Model file for the job. Use its own axes, mm. A direction names the side the tool comes from. Give positions to 0.01 mm unless a question says otherwise; leave off trailing zeros. Loops run counter-clockwise (first coordinate to the right, second up) from the corner with the lowest first, then second, coordinate; pieces in that order, holes last. Notation, with made-up numbers: M -8,-28.5 L -1,-28.5 A14 cw -1,-2.5 Z; hole C 87,-17 d4. An arc over 180 degrees is marked long. Answer in a Markdown table with one row per item.
```python
from build123d import *

# Parameters (mm, degrees)
F0_W      = 12.9794
F0_H      = 25.908
F1_DEPTH  = 25.4889
F2_W      = 38.1
F2_H      = 12.7
F3_DEPTH  = 6.35
F6_W      = 37.945812
F6_H      = 12.68057
F7_DEPTH  = 12.7
F8_W      = 50.9778
F8_H      = 12.7
F9_DEPTH  = 50.8
F10_R     = 12.7
F11_DEPTH = 12.701
F12_R     = 25.4


with BuildPart() as f1:
    # F0 (on Right) → F1 (new body, symmetric)
    with BuildSketch(Plane.YZ):
        with Locations((30.203413, 4.414101)):
            Rectangle(F0_W, F0_H)
    extrude(amount=F1_DEPTH, both=True)

    # F6 (on face) → F7 (join)
    with BuildSketch(Plane.XY.offset(17.368101)):
        with Locations((-6.515994, 30.352828)):
            Rectangle(F6_W, F6_H)
    extrude(amount=F7_DEPTH)

    # F8 (on face) → F9 (join)
    with BuildSketch(Plane(origin=(0, 36.693113, 0), x_dir=(-1, 0, 0), z_dir=(0, 1, 0))):
        with Locations((0, -2.189899)):
            Rectangle(F8_W, F8_H)
    extrude(amount=F9_DEPTH)

    # F10 (on face) → F11 (cut, through all)
    with BuildSketch(Plane.XY.offset(4.160101)):
        with Locations((-0.0889, 62.093113)):
            Circle(F10_R)
    extrude(amount=-F11_DEPTH, mode=Mode.SUBTRACT)

    # F12
    f12_edges = [f1.edges().sort_by_distance(p)[0] for p in [
        (-25.4889, 87.493113, -2.189899),
        (25.4889, 87.493113, -2.189899),
    ]]
    fillet(f12_edges, radius=F12_R)


with BuildPart() as f3:
    # F2 (on Front) → F3 (new body, symmetric)
    with BuildSketch(Plane.XZ):
        with Locations((6.389182, 23.830109)):
            Rectangle(F2_W, F2_H)
    extrude(amount=F3_DEPTH, both=True)


solid = f1.part
```
(1) Flat gauge pins, fed straight in: P1, Ø8, axis at x = 13.5, y = 50.5, coming from the +Z side; P2, Ø14, axis at y = 30, z = 26, coming from the +X side. Where does each tip first touch, or does it go through?
Established:
| item | result |
|---|---|
| P1 | stops at z = 4.16 |
| P2 | stops at x = 12.46 |
(2) Mould opens along X. For faces 4 (the flat face through (0, 36.693, 17)), 5 (the cylindrical face through (5.771, 50.826, -2.101)), 6 (the cylindrical face through (-17.85, 80.25, -2.1)), 7 (the flat face through (12.457, 30, 24)) say: pulls with the +X half, pulls with the -X half, needs draft (parallel to the pull), parting line crosses it, or undercut.
Established:
| item | result |
|---|---|
| face 4 | needs draft |
| face 5 | undercut |
| face 6 | pulls with the -X half |
| face 7 | pulls with the +X half |
(3) Saw through at B-B, the plane x = -6. Give the cut face in (y, z), and give its area (3 significant figures).
Established:
| item | result |
|---|---|
| outline | M 23.71,-8.54 L 50.85,-8.54 L 50.85,4.16 L 36.69,4.16 L 36.69,30.07 L 24.01,30.07 L 24.01,17.37 L 23.71,17.37 Z; M 73.33,-8.54 L 86.8,-8.54 L 86.8,4.16 L 73.33,4.16 Z |
| area | 848 mm2 |
(4) Which spindle directions (+Z, -Z, +X, -X, +Y, -Y) get a long thin tool onto all of the face, cutting with end or side? Do faces 1 (the cylindrical face through (18.2, 79.9, -2.1)), 2 (the flat face through (-7, 24.013, 24)), 3 (the flat face through (6, 50, 4.16)). Say none if no direction does.
Established:
| item | result |
|---|---|
| face 1 | +Z, -Z, +X, +Y |
| face 2 | +Z, +X, -X, -Y |
| face 3 | +Z, +X, -X, +Y |
(5) Saw through at A-A, the plane y = 64.5. Give the cut face in (x, z).
Established:
| item | result |
|---|---|
| outline | M -25.37,-8.54 L -12.56,-8.54 L -12.56,4.16 L -25.37,4.16 Z; M 12.38,-8.54 L 25.37,-8.54 L 25.37,4.16 L 12.38,4.16 Z |
(6) Saw through at D-D, the plane z = 12.5. Give the cut face in (x, y).
Established:
| item | result |
|---|---|
| outline | M -25.49,23.71 L 25.49,23.71 L 25.49,36.69 L -25.49,36.69 Z |
(7) Saw through at C-C, the plane y = 31. Give the cut face in (x, z), and give its area (3 significant figures).
Established:
| item | result |
|---|---|
| outline | M -25.49,-8.54 L 25.49,-8.54 L 25.49,17.37 L 12.46,17.37 L 12.46,30.07 L -25.49,30.07 Z |
| area | 1,800 mm2 |
(8) Wall check: L1, parallel to Y at x = 6.5, z = 26.5; L2, parallel to Z at x = -15.5, y = 73; L3, parallel to X at y = 28.5, z = 23.5. Give the ranges that are in metal, low to high.
Established:
| item | result |
|---|---|
| L1 | y = 24.01 to 36.69 |
| L2 | z = -8.54 to 4.16 |
| L3 | x = -25.49 to 12.46 |
